For this review, take the finished solid that the model builds, in its own axes (mm). A direction names the side the tool comes from. Coordinates: 2 decimals unless noted, no trailing zeros. Write each loop counter-clockwise with the first axis right and the second up, starting at its lowest first coordinate (ties: lowest second). Pieces come first, ordered by that corner, then holes. Notation, with made-up numbers: M 30.25,71.5 L 79.25,71.5 A27 ccw 79.25,98.5 Z; hole C -26,5.25 d10. An arc over 180 degrees is marked long. Return JSON: item names as keys, results as strings.
Autodesk Inventor part; units mm, degrees
ref_plane "YZ Plane" through (0, 0, 0) normal (1, 0, 0) x (0, 1, 0)
ref_plane "XZ Plane" through (0, 0, 0) normal (0, 1, 0) x (-1, 0, 0)
ref_plane "XY Plane" through (0, 0, 0) normal (0, 0, 1) x (1, 0, 0)
sketch "Sketch1" plane through (0, 0, 0) normal (0, 0, 1) x (1, 0, 0)
  line L0 (-4.19, 6.35) -> (4.19, 6.35)
  line L1 (4.19, 6.35) -> (4.19, -6.35)
  line L2 (4.19, -6.35) -> (-4.19, -6.35)
  line L3 (-4.19, -6.35) -> (-4.19, 6.35)
  line L4 (0, 0) -> (4.19, 0) construction
  line L5 (0, 0) -> (0, -6.35) construction
  dimension "d0" = 8.38
  dimension "d1" = 12.7
extrude "Extrusion1" add sketch "Sketch1" along normal blind 6.35
sketch "Sketch2" plane through (0, 0, 6.35) normal (0, 0, 1) x (1, 0, 0)
  line L0 (0, 0) -> (0, 14.132) construction
  line L1 (-2.075, 3.45) -> (2.075, 3.45)
  line L2 (2.075, 3.45) -> (2.075, -3.45)
  line L3 (2.075, -3.45) -> (-2.075, -3.45)
  line L4 (-2.075, -3.45) -> (-2.075, 3.45)
  line L5 (2.075, 0.15) -> (2.075, -3.45)
  line L6 (2.075, -3.45) -> (-2.075, -3.45)
  line L7 (-2.075, -3.45) -> (-2.075, 0.15)
  line L8 (0, 0) -> (4.19, 0) construction
  line L9 (4.19, -6.35) -> (4.19, 6.35) construction
  dimension "d4" = 4.15
  dimension "d20" = 6.9
extrude "Extrusion2" cut sketch "Sketch2" against normal blind 1
sketch "Sketch3" plane through (0, 0, 6.35) normal (0, 0, 1) x (1, 0, 0)
  line L0 (0, 0) -> (0, 14.132) construction
  line L1 (-1.905, 3.45) -> (1.905, 3.45)
  line L2 (1.905, 3.45) -> (1.905, -3.45)
  line L3 (1.905, -3.45) -> (-1.905, -3.45)
  line L4 (-1.905, -3.45) -> (-1.905, 3.45)
  line L5 (-1.905, -0.06) -> (1.905, -0.06)
  line L6 (1.905, -0.06) -> (1.905, -3.45)
  line L7 (1.905, -3.45) -> (-1.905, -3.45)
  line L8 (-1.905, -3.45) -> (-1.905, -0.06)
  line L9 (0, 0) -> (4.19, 0) construction
  line L10 (4.19, -6.35) -> (4.19, 6.35) construction
  line L11 (-2.075, 3.45) -> (2.075, 3.45)
  line L12 (2.075, -3.45) -> (-2.075, -3.45)
  point P0 (1.905, -0.06)
  dimension "d9" = 3.81
  dimension "d11" = 3.51
extrude "Extrusion3" add sketch "Sketch3" along normal blind 9.14 from surface at -6.35 contours L1 L2 L5 L4
sketch "Sketch4" plane through (-4.19, -6.35, 0) normal (0, -1, 0) x (1, 0, 0)
  line L0 (0, 0) -> (0, 6.35) construction
  line L1 (0, 3.175) -> (8.38, 3.175) construction
  line L2 (8.38, 0) -> (8.38, 6.35) construction
  line L3 (4.19, 0) -> (4.19, 6.35) construction
  line L4 (8.38, 6.35) -> (0, 6.35) construction
  line L5 (6.6, 4.445) -> (7.59, 4.445)
  line L6 (7.59, 4.445) -> (7.59, 1.905)
  line L7 (7.59, 1.905) -> (6.6, 1.905)
  line L8 (6.6, 1.905) -> (6.6, 4.445)
  line L9 (7.095, 4.445) -> (7.095, 1.905) construction
  line L10 (1.78, 4.445) -> (0.79, 4.445)
  line L11 (0.79, 4.445) -> (0.79, 1.905)
  line L12 (0.79, 1.905) -> (1.78, 1.905)
  line L13 (1.78, 1.905) -> (1.78, 4.445)
  line L14 (1.285, 4.445) -> (1.285, 1.905) construction
  dimension "d14" = 0.99
  dimension "d15" = 2.54
  dimension "d24" = 6.8
extrude "Extrusion4" add sketch "Sketch4" along normal blind 3.16
fillet "Fillet1" radius 0.51 4 edges at (-2.905, -9.51, 4.445) (-2.905, -9.51, 1.905) (2.905, -9.51, 4.445) (2.905, -9.51, 1.905)
equation "\"d7\" = switchTrackExtrusion"
equation "\"switchTrackExtrusion\" = 1"
properties part number "Switch_Base"
1. We need section D-D (x = -0.25). State the section outline as (y, z) points.
Checks:
{"outline": "M -6.35,0 L 6.35,0 L 6.35,6.35 L 3.45,6.35 L 3.45,9.14 L -0.06,9.14 L -0.06,5.35 L -3.45,5.35 L -3.45,6.35 L -6.35,6.35 Z"}
2. We need section B-B (y = -0.25). State the section outline as (x, z) points (3 decimals).
Checks:
{"outline": "M -4.19,0 L 4.19,0 L 4.19,6.35 L 2.075,6.35 L 2.075,5.35 L -2.075,5.35 L -2.075,6.35 L -4.19,6.35 Z"}
3. Draft analysis for pull direction X (two halves, no side actions). For faces 1 (the face through (-4.19, 0, 3)), 2 (the face through (0, -1, 5.35)), 3 (the face through (3, -9.51, 3)), state which applies: +X half, -X half, draft (parallel to the pull), parting line (faces both ways), or undercut.
Checks:
{"face 1": "-X half", "face 2": "undercut", "face 3": "draft"}
4. Clearance check with flat-ended pins moving along their axes: pin 1 Ø1.5 at (x, z) = (-1.5, 5.5) entering from -Y; pin 2 Ø2 at (x, y) = (3, -2) entering from -Z; pin 3 Ø2 at (y, z) = (-7.5, 4.5) entering from +X; pin 4 Ø1.1 at (y, z) = (2, 7.5) entering from -X (3 decimals). State where each tip first meets the part, or that it passes through.
Checks:
{"pin 1": "y = -6.35", "pin 2": "z = 0", "pin 3": "x = 3.4", "pin 4": "x = -1.905"}
5. We need section C-C (z = 2.75). State the section outline as (x, y) points.
Checks:
{"outline": "M -4.19,-6.35 L -3.4,-6.35 L -3.4,-9.51 L -2.41,-9.51 L -2.41,-6.35 L 2.41,-6.35 L 2.41,-9.51 L 3.4,-9.51 L 3.4,-6.35 L 4.19,-6.35 L 4.19,6.35 L -4.19,6.35 Z"}
6. For faces 4 (the face through (-3.4, -8, 3)), 5 (the face through (-1.905, 2, 7)), 6 (the face through (3, -8, 4.445)), 7 (the face through (3.4, -8, 3)), 8 (the face through (0, 3.45, 8)), list the 3-axis set-ups (+Z, -Z, +X, -X, +Y, -Y) from which the entire face can be reached by the end or side of a thin tool; tool diameter is ignored.
Checks:
{"face 4": "+Z, -Z, -X, -Y", "face 5": "+Z", "face 6": "+Z, +X, -X, -Y", "face 7": "+Z, -Z, +X, -Y", "face 8": "+Z, +X, -X, +Y"}
7. Wall thickness on L1, parallel to X at y = -8.5, z = 3.75; L2, parallel to Y at x = 1.75, z = 1; L3, parallel to Z at x = 3.25, y = -6.5 (3 decimals): over which ranges is each line inside the solid? List them lowest first. Write a range as from..to.
Checks:
{"L1": "-3.4..-2.41, 2.41..3.4", "L2": "-6.35..6.35", "L3": "1.905..4.445"}
8. We need section A-A (z = 5.75). State the section outline as (x, y) points (3 decimals).
Checks:
{"outline": "M -4.19,-6.35 L 4.19,-6.35 L 4.19,6.35 L -4.19,6.35 Z; hole M -2.075,-3.45 L 2.075,-3.45 L 2.075,3.45 L 1.905,3.45 L 1.905,-0.06 L -1.905,-0.06 L -1.905,3.45 L -2.075,3.45 Z"}
